Could you check a few things on this model? Use its own coordinates, in mm. A direction names the side the tool comes from. Give positions to 0.01 mm unless a question says otherwise; leave off trailing zeros. Order: outer loops, then holes, each group sorted by start corner. A loop starts at its lowest first (then second) coordinate and runs counter-clockwise, first axis right, second up.
(1) Imagine slicing it at C-C, the plane y = 3.5. Write out the boundary of the cut face in (x, z).
(2) If we mould it in two halves opening along Y, with no side actions, what happens to faces 6 (the cylindrical face through (3.46, 3.14, 11.1)), 7 (the cylindrical face through (0, 0, -5)), 8 (the cylindrical face through (-2.799, -0.176, 10.339))? For each: released by +Y, released by -Y, zero draft, split by the parting line, or undercut.
(3) Will these pins go through, and if not, where does the flat tip stop? pin 1 (4 mm diameter, centred on y = 0, z = -13, fed in from +X); pin 2 (0.6 mm diameter, centred on x = 5, y = 0, fed in from -Z); pin 3 (4.5 mm diameter, centred on y = 0, z = 9, fed in from +X).
(4) On a 3-axis mill with a long thin cutter (end or side, diameter ignored), from which of +Z, -Z, +X, -X, +Y, -Y can I reach the whole of each face in a straight line? I mean faces 1 (the flat face through (-6, -3, 9)), 2 (the flat face through (4, 0, 12)), 3 (the cylindrical face through (-3.54, -3.1, 11.14)), 4 (the flat face through (1, -0.9, 7.7)), 5 (the flat face through (5.014, -2.155, 10.268)). Say none if no direction works.
(5) If I drill on probe 1 along X at (y, z) = (1, 0); probe 2 along Z at (x, y) = (3, 0); probe 3 along Z at (x, y) = (-0.2, 0), over which ranges is the centre line in solid material (lowest first)?
(6) Imagine slicing it at B-B, the plane x = -3.25. Write out the boundary of the cut face in (y, z).
(7) Imagine slicing it at A-A, the plane z = 0. Write out the boundary of the cut face in (x, y), then the cut area to 3 significant figures.
from build123d import *

# Parameters (mm, degrees)
F1_DEPTH = 4
F2_R     = 1.35
F3_DEPTH = 25
F4_DEPTH = 2
F5_R     = 1.6
F6_DEPTH = 25
F7_SIZE  = 1.35
F8_R     = 3
F9_R     = 3.99999


# Not quite as in the source:
# - a fillet or chamfer is up to 0.001 mm smaller than in the source, because OpenCascade refuses the exact size
# - a feature names something its author has since deleted; it is built from what else it names


with BuildPart() as f1:
    # F0 (on Front) → F1 (new body, symmetric)
    with BuildSketch(Plane.XZ):
        with BuildLine():
            ThreePointArc((1, 4.8989794856), (0, -5), (-1, 4.8989794856))
            Line((-1, 4.8989794856), (-1, 12))
            Line((-1, 12), (-6, 12))
            Line((-6, 12), (-6, 5.2915026221))
            ThreePointArc((-6, 5.2915026221), (-7.6747647209, -2.257872113), (-2.1786734922, -7.6976218285))
            ThreePointArc((-2.1786734922, -7.6976218285), (-2.0136051919, -7.8104451764), (-1.95, -8))
            Line((-1.95, -8), (-1.95, -17))
            Line((-1.95, -17), (1.95, -17))
            Line((1.95, -17), (1.95, -8))
            ThreePointArc((1.95, -8), (2.0136051919, -7.8104451764), (2.1786734922, -7.6976218285))
            ThreePointArc((2.1786734922, -7.6976218285), (7.6747647209, -2.257872113), (6, 5.2915026221))
            Line((6, 5.2915026221), (6, 12))
            Line((6, 12), (1, 12))
            Line((1, 12), (1, 4.8989794856))
        make_face()
    extrude(amount=F1_DEPTH, both=True)

    # F2 (on face) → F3 (cut)
    with BuildSketch(Plane.YZ.offset(6)):
        with Locations((0, 9)):
            Circle(F2_R)
    extrude(amount=-F3_DEPTH, mode=Mode.SUBTRACT)

    # F2 (on face) → F4 (cut)
    with BuildSketch(Plane.YZ.offset(6)):
        Polygon((2.8867513459, 9), (1.443375673, 11.5), (-1.443375673, 11.5), (-2.8867513459, 9), (-1.443375673, 6.5), (1.443375673, 6.5), align=None)
        with Locations((0, 9)):
            Circle(F2_R, mode=Mode.SUBTRACT)
    extrude(amount=-F4_DEPTH, mode=Mode.SUBTRACT)

    # F5 (on face) → F6 (cut)
    with BuildSketch(Plane.YZ.offset(1.95)):
        with Locations((0, -13)):
            Circle(F5_R)
    extrude(amount=-F6_DEPTH, mode=Mode.SUBTRACT)

    # F7
    f7_edges = [f1.edges().sort_by_distance(p)[0] for p in [
        (-6, -1.35, 9),
    ]]
    chamfer(f7_edges, length=F7_SIZE)

    # F8
    f8_edges = [f1.edges().sort_by_distance(p)[0] for p in [
        (-3.5, -4, 12),
        (-3.5, 4, 12),
        (3.5, 4, 12),
        (3.5, -4, 12),
        (6, 0, 5.291503),
        (-6, 0, 5.291503),
    ]]
    fillet(f8_edges, radius=F8_R)

    # F9 (radius 4 in the source; OpenCascade refuses exactly that, so slightly less here)
    f9_edges = [f1.edges().sort_by_distance(p)[0] for p in [
        (0, -4, -17),
        (0, 4, -17),
    ]]
    fillet(f9_edges, radius=F9_R)


solid = f1.part
Answer block:
1. outline: (-6.55, 4.6) arc R8 ccw to (-2.18, -7.7) arc R0.31 cw to (-1.95, -8) - (-1.95, -14.94) - (1.95, -14.94) - (1.95, -8) arc R0.31 cw to (2.18, -7.7) arc R8 ccw to (6.55, 4.6) arc R3 cw to (6, 6.32) - (6, 10.66) - (1, 10.66) - (1, 4.9) arc R5 cw (long way) to (-1, 4.9) - (-1, 10.66) - (-6, 10.66) - (-6, 6.32) arc R3 cw to start
2. face 6: released by +Y
2. face 7: zero draft
2. face 8: undercut
3. pin 1: stops at x = 1.95
3. pin 2: stops at z = -6.47
3. pin 3: stops at x = 4
4. face 1: +Z, -X, +Y, -Y
4. face 2: +Z, +X, -X, +Y, -Y
4. face 3: +Z, +X, -X, -Y
4. face 4: +Z, +Y, -Y
4. face 5: +X
5. probe 1: x = -8 to -5, 5 to 8
5. probe 2: z = -7.42 to -4, 4 to 7.65, 10.35 to 12
5. probe 3: z = -17 to -14.6, -11.4 to -5
6. outline: (-4, -7.31) - (4, -7.31) - (4, -3.8) - (-4, -3.8) - close; (-4, 3.8) - (4, 3.8) - (4, 9) arc R3 ccw to (1, 12) - (-1, 12) arc R3 ccw to (-4, 9) - close; hole circle Ø2.7 at (0, 9)
7. outline: (-8, -4) - (-5, -4) - (-5, 4) - (-8, 4) - close; (5, -4) - (8, -4) - (8, 4) - (5, 4) - close
7. area: 48.0 mm2
